Study the drawing (mm; zero at the part's minimum x, y, z) and answer. A direction names the side the tool comes from. Round coordinates to 2 decimals unless told otherwise and drop trailing zeros. Loops run counter-clockwise (first coordinate to the right, second up) from the corner with the lowest first, then second, coordinate; pieces in that order, holes last. Notation, with made-up numbers: (-30, -14) - (3, -14) arc R11 cw to (3, -3) - close; hole circle Ø9 at (64.5, 65). An arc over 180 degrees is marked (long way). One line per item, written item: value.
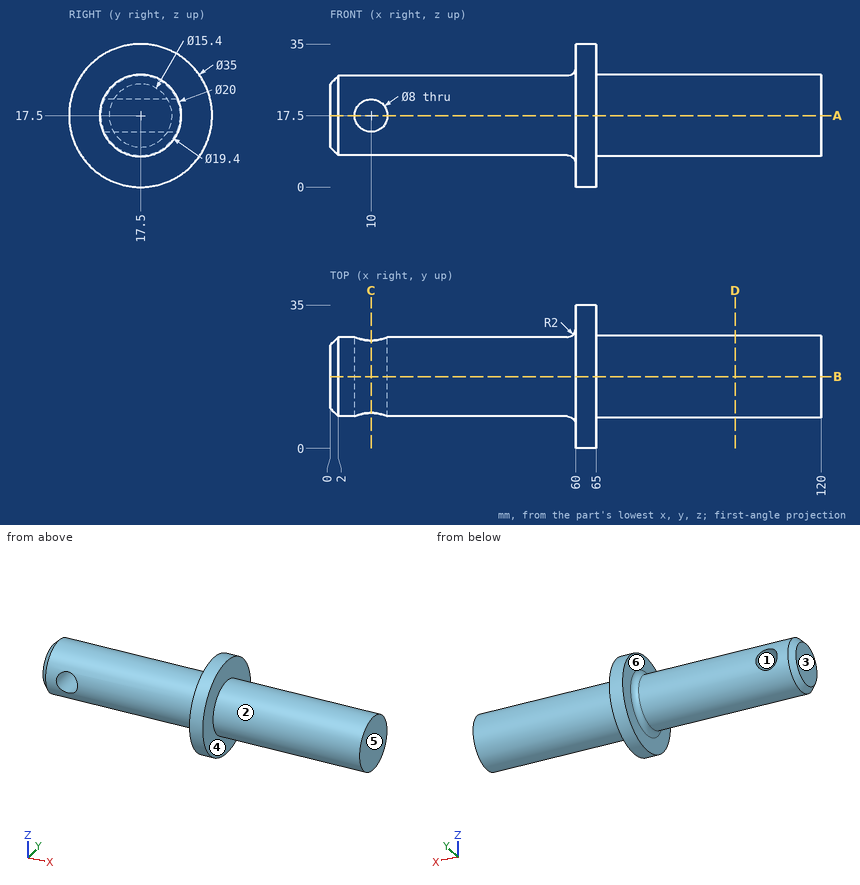
1) A cutting plane is placed at D-D on x = 99. Give the vertices of the cut face in (y, z).
Final values:
outline: circle Ø20 at (17.5, 17.5)
2) Consider L1, parallel to X at y = 22.5, z = 17.5; L2, parallel to X at y = 27, z = 18.5; L3, parallel to Z at x = 10, y = 23. Determine where each line is inside the solid, lowest interval first.
Final values:
L1: 0 to 6, 14 to 120
L2: 1.85 to 6.13, 13.87 to 120
L3: 9.51 to 13.5, 21.5 to 25.49
3) For a pull along Z with two mould halves and no side action, classify the marked faces 1, 2 and 3 as released by +Z, released by -Z, zero draft, split by the parting line, or undercut.
Final values:
face 1: undercut
face 2: split by the parting line
face 3: zero draft
4) For the marked faces 4, 5 and 6, determine the directions among +Z, -Z, +X, -X, +Y, -Y from which every point of the face is accessible in a straight line to the end or side of a thin tool.
Final values:
face 4: +X
face 5: +Z, -Z, +X, +Y, -Y
face 6: -X
5) A cutting plane is placed at A-A on z = 17.5. Give the vertices of the cut face in (x, y), and give its area (3 significant figures).
Final values:
outline: (0, 9.8) - (2, 7.8) - (6, 7.8) - (6, 27.2) - (2, 27.2) - (0, 25.2) - close; (14, 7.8) - (58, 7.8) arc R2 cw to (60, 5.8) - (60, 0) - (65, 0) - (65, 7.5) - (120, 7.5) - (120, 27.5) - (65, 27.5) - (65, 35) - (60, 35) - (60, 29.2) arc R2 cw to (58, 27.2) - (14, 27.2) - close
area: 2,280 mm2
6) Each of these flat-tipped pins is pushed along its axis until it touches: pin 1 Ø1 at (y, z) = (28.5, 4.5) entering from -X; pin 2 Ø4 at (x, y) = (85, 22.5) entering from +Z; pin 3 Ø4 at (y, z) = (18, 7) entering from -X; pin 4 Ø5 at (x, y) = (82, 4.5) entering from +Z. Where does it stop, or does it pass through?
Final values:
pin 1: x = 60
pin 2: z = 27.04
pin 3: x = 0.81
pin 4: through
7) A cutting plane is placed at B-B on y = 17.5. Give the vertices of the cut face in (x, z).
Final values:
outline: (0, 9.8) - (2, 7.8) - (58, 7.8) arc R2 cw to (60, 5.8) - (60, 0) - (65, 0) - (65, 7.5) - (120, 7.5) - (120, 27.5) - (65, 27.5) - (65, 35) - (60, 35) - (60, 29.2) arc R2 cw to (58, 27.2) - (2, 27.2) - (0, 25.2) - close; hole circle Ø8 at (10, 17.5)
8) A cutting plane is placed at C-C on x = 10. Give the vertices of the cut face in (y, z).
Final values:
outline: (8.66, 13.5) arc R9.7 ccw to (26.34, 13.5) - close; (8.66, 21.5) - (26.34, 21.5) arc R9.7 ccw to start
